Check sheet for the modelled part. Datum: model origin and axes. Units: mm. A direction names the side the tool comes from. Coordinates: 2 decimals unless noted, no trailing zeros. Write each loop counter-clockwise with the first axis right and the second up, starting at its lowest first coordinate (ties: lowest second). Pieces come first, ordered by that corner, then holes. Notation, with made-up numbers: (-10.5, 23) -> (-2.5, 23) arc R15 ccw to (-2.5, 40) -> close; hole circle Ø11 at (84.25, 0.25). An arc over 180 degrees is marked (long way). One line per item, written item: value. Start each with the question number.
1) Sectioned sample at C-C on x = -0.5. Enter the section's corners in (y, z).
2) Sectioned sample at A-A on x = -2. Enter the section's corners in (y, z), plus the area to 3 significant figures.
3) Gauge pin test, flat ends, axial feed: P1, Ø0.8, axis at y = 0, z = -11.5, coming from the +X side (3 decimals); P2, Ø1, axis at x = 0.5, z = -10.5, coming from the -Y side; P3, Ø3, axis at x = 1, y = 2.5, coming from the -Z side; P4, Ø3.5, axis at x = 0.5, y = -0.5, coming from the -Z side. Record the tip position at first contact, or that the pin passes through.
4) Scan lines: line 1 along Z through (x, y) = (2.5, 5.25); line 2 along Z through (x, y) = (-0.5, 2.5); line 3 along Y through (x, z) = (-0.5, 1.5). Record each from-to range of solid material in increasing order. Write a range as [from, to].
5) Draft check along Z on faces 6 (the flat face through (0, 0.38, -11)), 7 (the cylindrical face through (-0.439, 0.254, 13.321)). Enter one of: +Z half, -Z half, draft (parallel to the pull), parting line (faces both ways), or undercut.
6) Sectioned sample at B-B on z = 1. Enter the section's corners in (x, y) (3 decimals), plus the area to 3 significant figures.
7) Set-up check for faces 1 (the flat face through (1.5, 0.7, 8.89)), 2 (the flat face through (0, 5.08, -11)), 3 (the flat face through (0, -4.32, -11)), 4 (the flat face through (0, -5.08, -11)), 5 (the flat face through (3.43, 0, -4)): record each of +Z, -Z, +X, -X, +Y, -Y from which the full face is reachable in a straight line by a thin tool's end or side.
```python
from build123d import *

# Parameters (mm, degrees)
ESQUISSE1_W        = 6.86
ESQUISSE1_H        = 12.7
BOSS_EXTRU_1_DEPTH = 8.89
ESQUISSE2_R        = 3.175
BOSS_EXTRU_2_DEPTH = 8.89
ESQUISSE4_W        = 2.03
ESQUISSE4_H        = 0.76
BOSS_EXTRU_3_DEPTH = 3.96


with BuildPart() as part:
    # Esquisse1 → Boss.-Extru.1 (new body)
    with BuildSketch(Plane.XY):
        Rectangle(ESQUISSE1_W, ESQUISSE1_H)
    extrude(amount=-BOSS_EXTRU_1_DEPTH)

    # Esquisse2 → Boss.-Extru.2 (add)
    with BuildSketch(Plane.XY):
        with Locations(Location((0, 0, 0), (0, 0, 180))):
            Circle(ESQUISSE2_R)
    extrude(amount=BOSS_EXTRU_2_DEPTH)

    # Esquisse3 → Révolution1 (revolve)
    with BuildSketch(Plane(origin=(0, 0, 0), x_dir=(0, 0, -1), z_dir=(1, 0, 0))):
        with BuildLine():
            Line((-17.912911951, -0.906178747), (-8.89, 1.511503223))
            Line((-8.89, 1.511503223), (-8.512124194, 0.101251517))
            Line((-8.512124194, 0.101251517), (-18.945287852, -2.69430626))
            ThreePointArc((-18.945287852, -2.69430626), (-18.799433235, -1.586430454), (-17.912911951, -0.906178747))
        make_face()
    revolve(axis=Axis((0, 0, 8.89), (0, -0.2588190451025216, 0.9659258262890681)))

    # Esquisse4 → Boss.-Extru.3 (add)
    with BuildSketch(Plane(origin=(0, 0, -8.89), x_dir=(-1, 0, 0), z_dir=(0, 0, -1))):
        Rectangle(ESQUISSE4_W, ESQUISSE4_H)
        with Locations((0, 4.7)):
            Rectangle(ESQUISSE4_W, ESQUISSE4_H)
        with Locations((0, -4.7)):
            Rectangle(ESQUISSE4_W, ESQUISSE4_H)
    extrude(amount=BOSS_EXTRU_3_DEPTH)


solid = part.part
```
Answers:
1. outline: (-6.35, -8.89) -> (-5.08, -8.89) -> (-5.08, -12.85) -> (-4.32, -12.85) -> (-4.32, -8.89) -> (-0.38, -8.89) -> (-0.38, -12.85) -> (0.38, -12.85) -> (0.38, -8.89) -> (4.32, -8.89) -> (4.32, -12.85) -> (5.08, -12.85) -> (5.08, -8.89) -> (6.35, -8.89) -> (6.35, 0) -> (3.14, 0) -> (3.14, 8.89) -> (1.42, 8.89) -> (-0.99, 17.89) arc R1.37 ccw to (-3.64, 17.18) -> (-1.42, 8.89) -> (-3.14, 8.89) -> (-3.14, 0) -> (-6.35, 0) -> close
2. outline: (-6.35, -8.89) -> (6.35, -8.89) -> (6.35, 0) -> (2.47, 0) -> (2.47, 8.89) -> (-2.47, 8.89) -> (-2.47, 0) -> (-6.35, 0) -> close
2. area: 157 mm2
3. P1: stops at x = 1.015
3. P2: stops at y = -5.08
3. P3: stops at z = -8.89
3. P4: stops at z = -12.85
4. line 1: z = [-8.89, 0]
4. line 2: z = [-8.89, 8.89]
4. line 3: y = [-3.14, 3.14]
5. face 6: draft
5. face 7: undercut
6. outline: circle Ø6.35 at (0, 0)
6. area: 31.7 mm2
7. face 1: none
7. face 2: -Z, +X, -X, +Y
7. face 3: -Z, +X, -X
7. face 4: -Z, +X, -X, -Y
7. face 5: +Z, -Z, +X, +Y, -Y
